from build123d import *

# Parameters (mm, degrees)
SKETCH1_R           = 109.979208013
SKETCH1_R_2         = 55.789490447
BOSS_EXTRUDE1_DEPTH = 5
SKETCH1_3_R         = 55.789490447
BOSS_EXTRUDE2_DEPTH = 10
SKETCH1_4_W         = 5
SKETCH1_4_H         = 20
SKETCH1_4_H_2       = 30
CUT_EXTRUDE1_DEPTH  = 3
CIRPATTERN1_COUNT   = 12
SKETCH4_R           = 2.261632511
BOSS_EXTRUDE3_DEPTH = 8
CHAMFER1_SIZE2      = 2.331538291
CHAMFER1_SIZE       = 5


with BuildPart() as part:
    # Sketch1 → Boss-Extrude1 (new body)
    with BuildSketch(Plane(origin=(0, 0, 0), x_dir=(1, 0, 0), z_dir=(0, 1, 0))):
        with Locations(Location((0, 0, 0), (0, 0, 270))):
            Circle(SKETCH1_R)
        with Locations(Location((0, 0, 0), (0, 0, 270))):
            Circle(SKETCH1_R_2, mode=Mode.SUBTRACT)
    extrude(amount=-BOSS_EXTRUDE1_DEPTH)

    # Sketch1<3> → Boss-Extrude2 (add)
    with BuildSketch(Plane(origin=(0, 0, 0), x_dir=(1, 0, 0), z_dir=(0, 1, 0))):
        with Locations(Location((0, 0, 0), (0, 0, 270))):
            Circle(SKETCH1_3_R)
    extrude(amount=-BOSS_EXTRUDE2_DEPTH)

    # Sketch1<4> → Cut-Extrude1 (cut)
    with BuildSketch(Plane(origin=(0, 0, 0), x_dir=(1, 0, 0), z_dir=(0, 1, 0))):
        with Locations((0, 35)):
            Rectangle(SKETCH1_4_W, SKETCH1_4_H)
        with Locations((0, 78.089349727)):
            Rectangle(SKETCH1_4_W, SKETCH1_4_H_2)
    cut_extrude1 = extrude(amount=-CUT_EXTRUDE1_DEPTH, mode=Mode.SUBTRACT)

    # CirPattern1: Cut-Extrude1 ×12 about axis
    cirpattern1_axis = Axis((0, 0, 0), (0, 1, 0))
    for i in range(1, CIRPATTERN1_COUNT):
        add(cut_extrude1.rotate(cirpattern1_axis, i * 360 / CIRPATTERN1_COUNT), mode=Mode.SUBTRACT)

    # Sketch4 → Boss-Extrude3 (add)
    with BuildSketch(Plane.XY.offset(10)):
        with BuildLine():
            Line((-30.05733698, -10), (30.05733698, -10))
            Line((30.05733698, -10), (30.05733698, -10.774181914))
            ThreePointArc((30.05733698, -10.774181914), (0, -46.529878203), (-30.05733698, -10.774181914))
            Line((-30.05733698, -10.774181914), (-30.05733698, -10))
        make_face()
        with Locations((0, -26.625171413)):
            Circle(SKETCH4_R, mode=Mode.SUBTRACT)
    boss_extrude3 = extrude(amount=BOSS_EXTRUDE3_DEPTH)

    # Mirror1: Boss-Extrude3 across plane
    add(boss_extrude3.mirror(Plane.XY))

    # Chamfer1
    chamfer1_edges = [part.edges().sort_by_distance(p)[0] for p in [
        (0, -10, -55.789490447),
    ]]
    chamfer1_side = [part.faces().sort_by_distance(p)[0] for p in [
        (0, -9.953369234, -55.789490447),
    ]]
    chamfer(chamfer1_edges, length=CHAMFER1_SIZE - 0.0001, length2=CHAMFER1_SIZE2 - 0.0001, reference=chamfer1_side[0])  # a hair under: the kernel refuses the full size


solid = part.part
Work out the finished part from the listing and answer in its coordinate system (mm). A direction names the side the tool comes from. Give positions to 0.01 mm unless a question says otherwise; leave off trailing zeros. Write each loop counter-clockwise with the first axis right and the second up, starting at its lowest first coordinate (ties: lowest second). Pieces come first, ordered by that corner, then holes.
Q1. The part is cut by section C-C on z = -71.5. Give the vertices of the cut face in (x, y).
Answer:
outline: (-83.57, -5) - (83.57, -5) - (83.57, 0) - (44.17, 0) - (44.17, -3) - (38.39, -3) - (38.39, 0) - (2.5, 0) - (2.5, -3) - (-2.5, -3) - (-2.5, 0) - (-38.39, 0) - (-38.39, -3) - (-44.17, -3) - (-44.17, 0) - (-83.57, 0) - close
Q2. Given pin 1 (1 mm diameter, centred on x = 38, z = -8.5, fed in from -Y); pin 2 (1.5 mm diameter, centred on y = -1, z = 82.5, fed in from -X); pin 3 (1.5 mm diameter, centred on y = -2, z = 79.5, fed in from +X), each flat-ended and moving along its own axis, determine where each tip first touches the part or whether it passes through.
Answer:
pin 1: stops at y = -10
pin 2: stops at x = -73.57
pin 3: stops at x = 76.77
Q3. A tool of negligible diameter and unlimited length cuts with its end or side. For faces 1 (the face through (2, 0, -2)), 2 (the face through (-15.265, -1.479, 31.44)), 3 (the face through (0, -24, -10)), from which of +Z, -Z, +X, -X, +Y, -Y can it reach the whole face along a straight path? Write none if from no direction.
Answer:
face 1: +Z, -Z, +X, -X, +Y
face 2: +Y
face 3: +X, -X, -Y
Q4. The part is cut by section D-D on y = -18. Give the vertices of the cut face in (x, z).
Answer:
outline: (-30.45, -18) - (30.45, -18) - (30.45, -10) - (-30.45, -10) - close; (-30.45, 10) - (30.45, 10) - (30.45, 18) - (-30.45, 18) - close
Q5. The part is cut by section B-B on x = 75.5. Give the vertices of the cut face in (y, z).
Answer:
outline: (-5, -79.97) - (0, -79.97) - (0, -46.48) - (-3, -46.48) - (-3, -40.7) - (0, -40.7) - (0, -2.5) - (-3, -2.5) - (-3, 2.5) - (0, 2.5) - (0, 40.7) - (-3, 40.7) - (-3, 46.48) - (0, 46.48) - (0, 79.97) - (-5, 79.97) - close
Q6. The part is cut by section A-A on y = -41. Give the vertices of the cut face in (x, z), and give its area (3 significant figures).
Answer:
outline: (-17.52, -18) - (17.52, -18) - (17.52, -10) - (-17.52, -10) - close; (-17.52, 10) - (17.52, 10) - (17.52, 18) - (-17.52, 18) - close
area: 561 mm2
Q7. For a pull along Z with two mould halves and no side action, classify faces 4 (the face through (0, -24, 18)), 5 (the face through (92.735, -2.465, 59.124)), 6 (the face through (-68.695, -1.479, 36.775)) as released by +Z, released by -Z, zero draft, split by the parting line, or undercut.
Answer:
face 4: released by +Z
face 5: split by the parting line
face 6: undercut
Q8. Straight lines are drawn through the part: L1, parallel to Y at x = 0, z = -12; L2, parallel to Z at x = 22.5, y = -16.5; L3, parallel to X at y = -1.5, z = -16.5. For each, find the intervals that lie inside material, in ascending order.
Answer:
L1: y = -46.53 to -28.89, -24.36 to 0
L2: z = -18 to -10, 10 to 18
L3: x = -108.73 to -33.58, -23.58 to 23.58, 33.58 to 108.73
